Autodesk Inventor part; units mm, degrees
ref_plane "YZ Plane" through (0, 0, 0) normal (1, 0, 0) x (0, 1, 0)
ref_plane "XZ Plane" through (0, 0, 0) normal (0, 1, 0) x (-1, 0, 0)
ref_plane "XY Plane" through (0, 0, 0) normal (0, 0, 1) x (1, 0, 0)
sketch "スケッチ1" plane through (0, 0, 0) normal (0, 0, 1) x (1, 0, 0)
  line L0 (-12.5, 25) -> (12.5, 25)
  line L1 (12.5, 25) -> (12.5, -25)
  line L2 (12.5, -25) -> (-12.5, -25)
  line L3 (-12.5, -25) -> (-12.5, 25)
  line L4 (-10.5, 23) -> (10.5, 23)
  line L5 (10.5, 23) -> (10.5, -23)
  line L6 (10.5, -23) -> (-10.5, -23)
  line L7 (-10.5, -23) -> (-10.5, 23)
  point P0 (0, 0)
  dimension "d0" = 25
  dimension "d1" = 50
  dimension "d2" = 46
  dimension "d3" = 21
  dimension "d4" = 25
  dimension "d5" = 23
  dimension "d6" = 10.5
  dimension "d7" = 12.5
extrude "押し出し1" add sketch "スケッチ1" along normal blind 60
sketch "スケッチ2" plane through (-12.5, 25, 0) normal (0, 1, 0) x (1, 0, 0)
  line L0 (0, 0) -> (25, 0)
  line L1 (0, 0) -> (0, -60)
  arc A0 (6, -33.5) -> (19, -33.5) centre (12.5, -33.5) ccw
  line L2 (6, -33.5) -> (6, 0)
  line L3 (19, -33.5) -> (19, 0)
  point P0 (12.5, 0)
  dimension "d10" = 13
  dimension "d11" = 33.5
  dimension "d12" = 12.5
extrude "押し出し2" cut sketch "スケッチ2" against normal blind 2
sketch "スケッチ3" plane through (-12.5, 25, 60) normal (0, 1, 0) x (1, 0, 0)
  arc A0 (6, 26.5) -> (19, 26.5) centre (12.5, 26.5) ccw
  circle A1 centre (4.5, 20) radius 1
  circle A2 centre (4.5, 56) radius 1
  circle A3 centre (20.5, 56) radius 1
  circle A4 centre (20.5, 20) radius 1
  point P0 (12.5, 60)
  dimension "d15" = 6.5
  dimension "d16" = 6.5
  dimension "d17" = 2
  dimension "d18" = 8
  dimension "d19" = 8
  dimension "d20" = 8
  dimension "d21" = 8
  dimension "d22" = 29.5
  dimension "d23" = 29.5
hole "穴1" at (-8, 25, 4) at (8, 25, 4) at (8, 25, 40) at (-8, 25, 40) direction (0, -1, 0) diameter 2 depth 2 tip angle 118 counterbore diameter 4 counterbore depth 0.5
sketch "スケッチ4" plane through (-12.5, -25, 0) normal (0, -1, 0) x (1, 0, 0)
  line L0 (25, 0) -> (0, 0)
  line L1 (25, 0) -> (25, 60)
  circle A0 centre (12.5, 10.5) radius 2
  point P0 (12.5, 0)
  dimension "d31" = 4
  dimension "d32" = 12.5
  dimension "d33" = 10.5
hole "穴2" at (0, -25, 10.5) direction (0, 1, 0) diameter 4 end through all
sketch "スケッチ5" plane through (-12.5, 25, 60) normal (0, 1, 0) x (1, 0, 0)
  line L0 (0, 0) -> (25, 0)
  arc A0 (6, 26.5) -> (19, 26.5) centre (12.5, 26.5) ccw
  circle A1 centre (20.5, 4) radius 1.5
  circle A2 centre (4.5, 4) radius 1.5
  point P0 (12.5, 60)
  dimension "d43" = 4
  dimension "d44" = 4
  dimension "d46" = 8
  dimension "d47" = 8
  dimension "d57" = 3
hole "穴4" at (-8, 25, 56) at (8, 25, 56) direction (0, -1, 0) diameter 3 end through all
thread "ねじ1"
thread "ねじ2"
thread "ねじ3"
thread "ねじ4"
properties part number "10" material "アルミニウム 6061"
Work out the finished part from the listing and answer in its coordinate system (mm). A direction names the side the tool comes from. Coordinates: 2 decimals unless noted, no trailing zeros. Write each loop counter-clockwise with the first axis right and the second up, starting at its lowest first coordinate (ties: lowest second). Pieces come first, ordered by that corner, then holes.
1. The part is cut by section D-D, the plane z = 56. Write down the section's boundary in (x, y), and give its area (3 significant figures).
Results list:
outline: (-12.5, -25) - (-9.5, -25) - (-9.5, -23) - (-10.5, -23) - (-10.5, 23) - (-9.5, 23) - (-9.5, 25) - (-12.5, 25) - close; (-6.5, -25) - (6.5, -25) - (6.5, -23) - (-6.5, -23) - close; (-6.5, 23) - (6.5, 23) - (6.5, 25) - (-6.5, 25) - close; (9.5, -25) - (12.5, -25) - (12.5, 25) - (9.5, 25) - (9.5, 23) - (10.5, 23) - (10.5, -23) - (9.5, -23) - close
area: 260 mm2
2. The part is cut by section B-B, the plane y = 6.5. Write down the section's boundary in (x, z).
Results list:
outline: (-12.5, 0) - (-10.5, 0) - (-10.5, 60) - (-12.5, 60) - close; (10.5, 0) - (12.5, 0) - (12.5, 60) - (10.5, 60) - close
3. The part is cut by section A-A, the plane x = -8. State how many separate pieces and enclosed holes the cut face has, and give its area (3 significant figures).
Results list:
separate pieces: 6
enclosed holes: 0
area: 218 mm2
4. Flat-ended cylindrical pins translate along their axes: pin 1 (3 mm diameter, centred on x = 0, z = 10.5, fed in from -Y); pin 2 (2 mm diameter, centred on x = 7.5, z = 39.5, fed in from +Y). Find the tip coordinate at first contact, or state that the pin passes through.
Results list:
pin 1: passes through
pin 2: stops at y = 24.5
5. The part is cut by section C-C, the plane z = 4. Write down the section's boundary in (x, y).
Results list:
outline: (-12.5, -25) - (12.5, -25) - (12.5, 25) - (10, 25) - (10, 24.5) - (9, 24.5) - (9, 23) - (10.5, 23) - (10.5, -23) - (-10.5, -23) - (-10.5, 23) - (-9, 23) - (-9, 24.5) - (-10, 24.5) - (-10, 25) - (-12.5, 25) - close; (-7, 23) - (-6.5, 23) - (-6.5, 24.5) - (-7, 24.5) - close; (6.5, 23) - (7, 23) - (7, 24.5) - (6.5, 24.5) - close
6. For faces 3 (the cylindrical face through (0, 24, 40)), 4 (the flat face through (-7, 23, 36)), 5 (the cylindrical face through (10, 24.75, 3.93)), determine the directions among +Z, -Z, +X, -X, +Y, -Y from which every point of the face is accessible in a straight line to the end or side of a thin tool.
Results list:
face 3: -Z, +Y
face 4: +Z, -Z
face 5: +Y
7. Consider line 1 along Z through (x, y) = (8, 23.8); line 2 along X through (y, z) = (-24.6, 56); line 3 along X through (y, z) = (20, 17.5). Determine where each line is inside the solid, lowest interval first.
Results list:
line 1: z = 0 to 3, 5 to 39, 41 to 54.5, 57.5 to 60
line 2: x = -12.5 to -9.5, -6.5 to 6.5, 9.5 to 12.5
line 3: x = -12.5 to -10.5, 10.5 to 12.5
8. For a pull along X with two mould halves and no side action, classify faces 1 (the flat face through (-11, -2, 0)), 2 (the cylindrical face through (8, 24, 41)) as +X half, -X half, draft (parallel to the pull), parting line (faces both ways), or undercut.
Results list:
face 1: draft
face 2: undercut
